CAD build for the part. Positions are in the model's coordinates, mm. Face numbers are marked on the shaded views. A direction names the side the tool comes from. Coordinates: 2 decimals unless noted, no trailing zeros. Order: outer loops, then holes, each group sorted by start corner. A loop starts at its lowest first (then second) coordinate and runs counter-clockwise, first axis right, second up. Notation, with made-up numbers: (5, -18) - (45, -18) arc R27 cw to (45, 5) - close; hole circle Ø7 at (79.5, 11). An arc over 180 degrees is marked (long way). Write each question's results on one line, items separated by ' | '. Start each with the question number.
Q1. Band-saw the part on B-B, the plane y = -9.25. Write the cut outline in (x, z).
Q2. Which spindle directions (+Z, -Z, +X, -X, +Y, -Y) get a long thin tool onto all of the face, cutting with end or side? Do the marked faces 1, 2, 3 and 4. Say none if no direction does.
Q3. Band-saw the part on D-D, the plane y = -17.75. Write the cut outline in (x, z), then the cut area to 3 significant figures.
Q4. Pin check, flat tips, straight feed: P1, Ø0.5, axis at x = 3, y = -19.5, coming from the +Z side; P2, Ø4, axis at x = -1, z = 35.5, coming from the +Y side; P3, Ø5.5, axis at x = 0, z = 45, coming from the -Y side; P4, Ø6, axis at y = -3, z = 40.5, coming from the +X side. Stop position of each tip, or through.
Q5. Band-saw the part on A-A, the plane z = 45. Write the cut outline in (x, y).
Q6. Pull direction Y, two halves, no side cores. Call the marked faces 5, 6 and 7: released by +Y, released by -Y, zero draft, split by the parting line, or undercut.
Q7. Wall check: probe 1 along X at (y, z) = (-20.5, 46.5); probe 2 along Y at (x, z) = (-6.4, 45); probe 3 along X at (y, z) = (-5.5, 40.5). Give the ranges that are in metal, low to high.
Q8. Band-saw the part on C-C, the plane x = 2.25. Write the cut outline in (y, z), then the cut area to 3 significant figures.
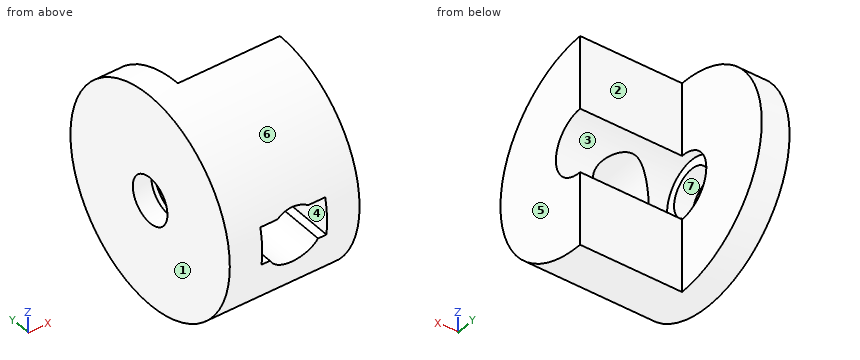
```python
from build123d import *

# Parameters (mm, degrees)
SKETCH054_R     = 11.5
PAD018_DEPTH    = 14
SKETCH055_W     = 11.5
SKETCH055_H     = 23
POCKET033_DEPTH = 11
SKETCH056_R     = 3
POCKET034_DEPTH = 11.501
SKETCH057_R     = 2.5
POCKET035_DEPTH = 3
SKETCH058_R     = 3.5
POCKET036_DEPTH = 12
SKETCH059_W     = 7
SKETCH059_H     = 4
POCKET037_DEPTH = 8


with BuildPart() as part:
    # Sketch054 → Pad018 (new body)
    with BuildSketch(Plane.YZ):
        with Locations((-11, 45)):
            Circle(SKETCH054_R)
    extrude(amount=PAD018_DEPTH)

    # Sketch055 (on Face3 of Pad018) → Pocket033 (cut)
    with BuildSketch(Plane.YZ.offset(14)):
        with Locations((-5.25, 45)):
            Rectangle(SKETCH055_W, SKETCH055_H)
    extrude(amount=-POCKET033_DEPTH, mode=Mode.SUBTRACT)

    # Sketch056 (on Face4 of Pocket033) → Pocket034 (cut, through all)
    with BuildSketch(Plane.ZX.offset(-11)):
        with Locations((45, 7)):
            Circle(SKETCH056_R)
    extrude(amount=-POCKET034_DEPTH, mode=Mode.SUBTRACT)

    # Sketch057 (on Face5 of Pocket034) → Pocket035 (cut)
    with BuildSketch(Plane(origin=(0, 0, 0), x_dir=(0, 1, 0), z_dir=(-1, 0, 0))):
        with Locations((-11, -45)):
            Circle(SKETCH057_R)
    extrude(amount=-POCKET035_DEPTH, mode=Mode.SUBTRACT)

    # Sketch058 (on Face4 of Pocket035) → Pocket036 (cut)
    with BuildSketch(Plane.YZ.offset(14)):
        with Locations((-11, 45)):
            Circle(SKETCH058_R)
    extrude(amount=-POCKET036_DEPTH, mode=Mode.SUBTRACT)

    # Sketch059 → Pocket037 (cut)
    with BuildSketch(Plane.XZ.offset(25)):
        with Locations((7, 45.5)):
            Rectangle(SKETCH059_W, SKETCH059_H)
    extrude(amount=-POCKET037_DEPTH, mode=Mode.SUBTRACT)


with BuildPart() as part_1:
    # Body004 placement: moved
    add(part.part.moved(Location((-7, 0, 0))))


solid = part_1.part
```
Results below:
1) outline: (-7, 33.63) - (-4, 33.63) - (-4, 41.97) - (-5, 41.97) - (-5, 43.21) - (-7, 43.21) - close; (-7, 46.79) - (-5, 46.79) - (-5, 48.03) - (-4, 48.03) - (-4, 56.37) - (-7, 56.37) - close
2) face 1: +Z, -Z, -X, +Y, -Y | face 2: +Z, -Z, +X, +Y | face 3: +X | face 4: -Y
3) outline: (-7, 35.69) - (7, 35.69) - (7, 54.31) - (-7, 54.31) - close; hole (-3.5, 43.5) - (-2.6, 43.5) arc R3 ccw to (2.6, 43.5) - (3.5, 43.5) - (3.5, 47.5) - (1.66, 47.5) arc R3 ccw to (-1.66, 47.5) - (-3.5, 47.5) - close | area: 226 mm²
4) P1: stops at z = 53.01 | P2: stops at y = -11 | P3: passes through | P4: stops at x = -4
5) outline: (-7, -22.5) - (-3.5, -22.5) - (-3.5, -17) - (-3, -17) - (-3, -14.5) - (-5, -14.5) - (-5, -13.5) - (-7, -13.5) - close; (-7, -8.5) - (-5, -8.5) - (-5, -7.5) - (-4, -7.5) - (-4, 0.5) - (-7, 0.5) - close; (3, -17) - (3.5, -17) - (3.5, -22.5) - (7, -22.5) - (7, -14.5) - (3, -14.5) - close
6) face 5: zero draft | face 6: split by the parting line | face 7: undercut
7) probe 1: x = -7 to -3.5, 3.5 to 7 | probe 2: y = -22.5 to -13.5, -8.5 to 0.5 | probe 3: x = -7 to -4
8) outline: (-22.33, 43.02) arc R11.5 ccw to (-11, 33.5) - (-11, 41.5) arc R3.5 cw to (-13.88, 43.02) - close; (-22.22, 47.5) - (-17, 47.5) - (-17, 46.98) - (-13.88, 46.98) arc R3.5 cw to (-11, 48.5) - (-11, 56.5) arc R11.5 ccw to start | area: 153 mm²
